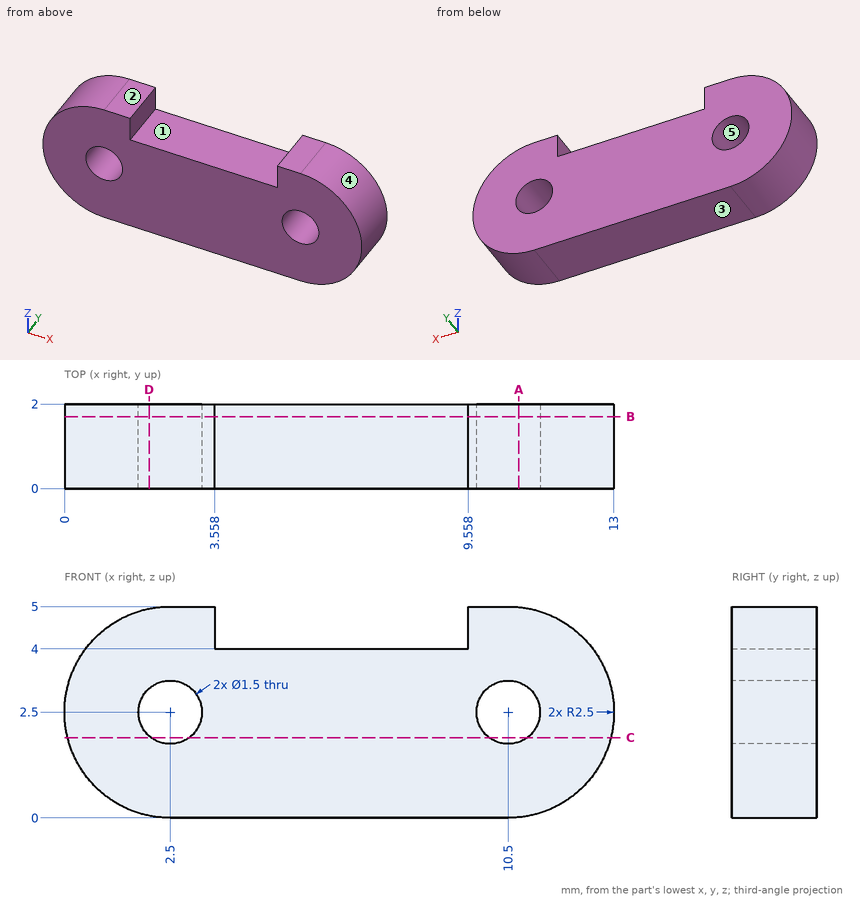
Source: three-view drawing plus pictorial views. Frame: mm from the lowest corner of the part. A direction names the side the tool comes from. Round coordinates to 2 decimals unless told otherwise and drop trailing zeros. Loops run counter-clockwise (first coordinate to the right, second up) from the corner with the lowest first, then second, coordinate; pieces in that order, holes last.
1. Section query A-A on x = 10.75. Output: boundary loops of the cut face in (y, z), and give its area (3 significant figures).
2. Section query C-C on z = 1.9. Output: boundary loops of the cut face in (x, y).
3. Mould query, pull axis X, two halves, no side actions, for the marked faces 3, 4 and 5. Classes: released by +X, released by -X, zero draft, split by the parting line, or undercut.
4. Section query B-B on y = 1.7. Output: boundary loops of the cut face in (x, z), and give its area (3 significant figures).
5. Ray query, L1, parallel to Z at x = 2.5, y = 0.8; L2, parallel to Z at x = 6, y = 1.65; L3, parallel to X at y = 0.45, z = 4.1. Return the intervals inside material, ascending.
6. Access query for the marked faces 1 and 2. Directions: +Z, -Z, +X, -X, +Y, -Y. A direction counts if a zero-diameter tool reaches every point of the face in a straight line with its end or side. Return the directions, or none.
7. Contact query for flat-ended pins moving along their axis: pin 1 (0.5 mm diameter, centred on y = 1.5, z = 4.5, fed in from -X) (1 decimal); pin 2 (0.6 mm diameter, centred on x = 5.5, y = 0.5, fed in from +Z); pin 3 (0.8 mm diameter, centred on y = 1, z = 4.5, fed in from +X). Output: stop coordinate, or through.
8. Section query D-D on x = 2. Output: boundary loops of the cut face in (y, z).
Answers below:
1. outline: (0, 0.01) - (2, 0.01) - (2, 1.79) - (0, 1.79) - close; (0, 3.21) - (2, 3.21) - (2, 4.99) - (0, 4.99) - close
1. area: 7.12 mm2
2. outline: (0.07, 0) - (2.05, 0) - (2.05, 2) - (0.07, 2) - close; (2.95, 0) - (10.05, 0) - (10.05, 2) - (2.95, 2) - close; (10.95, 0) - (12.93, 0) - (12.93, 2) - (10.95, 2) - close
3. face 3: zero draft
3. face 4: released by +X
3. face 5: undercut
4. outline: (2.5, 0) - (10.5, 0) arc R2.5 ccw to (10.5, 5) - (9.56, 5) - (9.56, 4) - (3.56, 4) - (3.56, 5) - (2.5, 5) arc R2.5 ccw to start; hole circle Ø1.5 at (2.5, 2.5); hole circle Ø1.5 at (10.5, 2.5)
4. area: 50.1 mm2
5. L1: z = 0 to 1.75, 3.25 to 5
5. L2: z = 0 to 4
5. L3: x = 0.58 to 3.56, 9.56 to 12.42
6. face 1: +Z, +Y, -Y
6. face 2: +Z, +X, -X, +Y, -Y
7. pin 1: stops at x = 0.7
7. pin 2: stops at z = 4
7. pin 3: stops at x = 12.42
8. outline: (0, 0.05) - (2, 0.05) - (2, 1.94) - (0, 1.94) - close; (0, 3.06) - (2, 3.06) - (2, 4.95) - (0, 4.95) - close
